from build123d import *
from OCP.BRepFilletAPI import BRepFilletAPI_MakeChamfer

# Parameters (mm, degrees)
CROQUIS2_W              = 16
CROQUIS2_H              = 23
SALIENTE_EXTRUIR1_DEPTH = 6
CORTAR_EXTRUIR1_DEPTH   = 3
CHAFL_N2_SIZE           = 3
CHAFL_N2_SIZE2          = 3.575260778
REDONDEO1_R             = 10
CHAFL_N1_SIZE           = 1
CROQUIS4_W              = 16
CROQUIS4_H              = 7
CORTAR_EXTRUIR2_DEPTH   = 1
SALIENTE_EXTRUIR2_DEPTH = 7
MATRIZL1_COUNT          = 8
MATRIZL1_PITCH          = 2


with BuildPart() as part:
    # Croquis2 → Saliente-Extruir1 (new body)
    with BuildSketch(Plane(origin=(0, 0, 0), x_dir=(-1, 0, 0), z_dir=(0, 0, -1))):
        with Locations((-8, 11.5)):
            Rectangle(CROQUIS2_W, CROQUIS2_H)
        with BuildLine():
            Line((-9.977670702, 6.125), (-9.977670702, 4.875))
            Line((-9.977670702, 4.875), (-9.124878317, 4.159422225))
            ThreePointArc((-9.124878317, 4.159422225), (-6.25, 5.5), (-9.124878317, 6.840577775))
            Line((-9.124878317, 6.840577775), (-9.977670702, 6.125))
        make_face(mode=Mode.SUBTRACT)
        with BuildLine():
            Line((-9.977670702, 18.125), (-9.977670702, 16.875))
            Line((-9.977670702, 16.875), (-9.124878317, 16.159422225))
            ThreePointArc((-9.124878317, 16.159422225), (-6.25, 17.5), (-9.124878317, 18.840577775))
            Line((-9.124878317, 18.840577775), (-9.977670702, 18.125))
        make_face(mode=Mode.SUBTRACT)
    extrude(amount=SALIENTE_EXTRUIR1_DEPTH)

    # Croquis3 → Cortar-Extruir1 (cut)
    with BuildSketch(Plane(origin=(-8, 0, 0), x_dir=(-1, 0, 0), z_dir=(0, 0, -1))):
        with BuildLine():
            Line((-19.864348845, 6.5), (-19.864348845, 4.5))
            Line((-19.864348845, 4.5), (-18.089059731, 3.01035556))
            ThreePointArc((-18.089059731, 3.01035556), (-12.75, 5.5), (-18.089059731, 7.98964444))
            Line((-18.089059731, 7.98964444), (-19.864348845, 6.5))
        make_face()
        with BuildLine():
            Line((-19.864348845, 18.5), (-18.089059731, 19.98964444))
            ThreePointArc((-18.089059731, 19.98964444), (-12.75, 17.5), (-18.089059731, 15.01035556))
            Line((-18.089059731, 15.01035556), (-19.864348845, 16.5))
            Line((-19.864348845, 16.5), (-19.864348845, 18.5))
        make_face()
    extrude(amount=CORTAR_EXTRUIR1_DEPTH, mode=Mode.SUBTRACT)

    # Chaflán2: one chamfer whose edges measure the first distance from different faces: ONE call of the kernel's chamfer builder (chamfer() names one face for all edges)
    chafl_n2_edges_1 = [part.edges().sort_by_distance(p)[0] for p in [
        (16, 23, -3),
        (16, 0, -3),
    ]]
    chafl_n2_side_1 = [part.faces().sort_by_distance(p)[0] for p in [
        (16, 11.5, -3),
    ]]
    chafl_n2_edges_2 = [part.edges().sort_by_distance(p)[0] for p in [
        (0, 23, -3),
        (0, 0, -3),
    ]]
    chafl_n2_side_2 = [part.faces().sort_by_distance(p)[0] for p in [
        (0, 11.5, -3),
    ]]
    chafl_n2 = BRepFilletAPI_MakeChamfer(part.part.solid().wrapped)
    for e in chafl_n2_edges_1:
        chafl_n2.Add(CHAFL_N2_SIZE, CHAFL_N2_SIZE2, e.wrapped, chafl_n2_side_1[0].wrapped)  # the first distance lies on this face
    for e in chafl_n2_edges_2:
        chafl_n2.Add(CHAFL_N2_SIZE, CHAFL_N2_SIZE2, e.wrapped, chafl_n2_side_2[0].wrapped)  # the first distance lies on this face
    add(Compound.cast(chafl_n2.Shape()), mode=Mode.REPLACE)

    # Redondeo1
    redondeo1_edges = [part.edges().sort_by_distance(p)[0] for p in [
        (3.575260778, 23, -3),
        (12.424739222, 23, -3),
        (3.575260778, 0, -3),
        (12.424739222, 0, -3),
    ]]
    fillet(redondeo1_edges, radius=REDONDEO1_R)

    # Chaflán1
    chafl_n1_edges = [part.edges().sort_by_distance(p)[0] for p in [
        (8, 0, 0),
        (8, 23, 0),
        (0.393543512, 20.330222216, 0),
        (15.606456488, 2.669777784, 0),
        (3.794761687, 22.396926208, 0),
        (12.205238313, 22.396926208, 0),
        (12.205238313, 0.603073792, 0),
        (3.794761687, 0.603073792, 0),
        (16, 11.5, 0),
        (0, 11.5, 0),
        (0.393543512, 2.669777784, 0),
        (15.606456488, 20.330222216, 0),
    ]]
    chamfer(chafl_n1_edges, length=CHAFL_N1_SIZE)

    # Croquis4 → Cortar-Extruir2 (cut)
    with BuildSketch(Plane(origin=(0, 0, -6), x_dir=(-1, 0, 0), z_dir=(0, 0, -1))):
        with Locations((-8, 11.5)):
            Rectangle(CROQUIS4_W, CROQUIS4_H)
    extrude(amount=-CORTAR_EXTRUIR2_DEPTH, mode=Mode.SUBTRACT)

    # Croquis5 → Saliente-Extruir2 (add)
    with BuildSketch(Plane(origin=(0, 8, 0), x_dir=(1, 0, 0), z_dir=(0, 1, 0))):
        Polygon((0, 5), (0.839099631, 6), (1.25, 6), (1.25, 5), align=None)
    saliente_extruir2 = extrude(amount=SALIENTE_EXTRUIR2_DEPTH)

    # MatrizL1: Saliente-Extruir2 ×8
    with Locations(*[(i * MATRIZL1_PITCH, 0, 0) for i in range(1, MATRIZL1_COUNT)]):
        add(saliente_extruir2)


solid = part.part
Input: part model. Units: mm. Frame: model coordinates. A direction names the side the tool comes from. Coordinates: 2 decimals unless noted, no trailing zeros. Loops run counter-clockwise (first coordinate to the right, second up) from the corner with the lowest first, then second, coordinate; pieces in that order, holes last. Notation, with made-up numbers: (62, 8) - (79, 8) arc R35 cw to (79, 41) - close; hole circle Ø10 at (64.5, 2.25). An arc over 180 degrees is marked (long way). Answer in a Markdown table with one row per item. Add a question column.
Item 1: Line query: line 1 along Y through (x, z) = (8, -4.2); line 2 along Y through (x, z) = (8, -1.75); line 3 along X through (y, z) = (5.5, -1.5). Output: solid intervals per line, ascending. Write a range as [from, to].
Item 2: Section query D-D on z = -5.5. State how many separate pieces and enclosed holes the cut face has, then the cut area to 3 significant figures.
Item 3: Access query for faces 5 (the flat face through (0, 11, -3)), 6 (the flat face through (13.9, 8, -5.6)), 7 (the cylindrical face through (4.75, 17.6, -1.48)). Directions: +Z, -Z, +X, -X, +Y, -Y. A direction counts if a zero-diameter tool reaches every point of the face in a straight line with its end or side. Return the directions, or none.
Item 4: Section query B-B on z = -2.25. Return the cut outline in (x, y), then the cut area to 3 significant figures.
Item 5: Contact query for flat-ended pins moving along their axis: P1, Ø1, axis at x = 12.5, z = -3, coming from the -Y side; P2, Ø2, axis at x = 12.5, z = -3.5, coming from the +Y side; P3, Ø0.6, axis at x = 15.5, z = -5.5, coming from the -Y side. Output: stop coordinate, or through.
Item 6: Section query C-C on z = -3.5. Return the cut outline in (x, y) (3 decimals).
Item 7: Section query A-A on y = 5.5. Return the cut outline in (x, z).
Item 8: Mould query, pull axis Y, two halves, no side actions, for faces 1 (the flat face through (0.2, 8, -5.7)), 2 (the flat face through (8.41, 11.45, -5.49)), 3 (the cylindrical face through (3.8, 22.4, -3.5)), 4 (the conical face through (4.045, 1.155, -0.396)). Classes: released by +Y, released by -Y, zero draft, split by the parting line, or undercut.
Recorded:
| question | item | result |
|---|---|---|
| 1 | line 1 | [0, 3.75], [7.25, 15.75], [19.25, 23] |
| 1 | line 2 | [0, 2.25], [8.75, 14.25], [20.75, 23] |
| 1 | line 3 | [0, 4.75], [11.86, 16] |
| 2 | separate pieces | 1 |
| 2 | enclosed holes | 9 |
| 2 | area | 255 mm^2 |
| 3 | face 5 | +Z, -Z, -X, +Y, -Y |
| 3 | face 6 | -Z |
| 3 | face 7 | +Z |
| 4 | outline | (0, 3) - (0.79, 2.34) arc R10 ccw to (7.21, 0) - (8.79, 0) arc R10 ccw to (15.21, 2.34) - (16, 3) - (16, 20) - (15.21, 20.66) arc R10 ccw to (8.79, 23) - (7.21, 23) arc R10 ccw to (0.79, 20.66) - (0, 20) - close; hole (10.09, 3.01) - (11.86, 4.5) - (11.86, 6.5) - (10.09, 7.99) arc R3.25 ccw (long way) to start; hole (10.09, 15.01) - (11.86, 16.5) - (11.86, 18.5) - (10.09, 19.99) arc R3.25 ccw (long way) to start |
| 4 | area | 270 mm^2 |
| 5 | P1 | y = 0.53 |
| 5 | P2 | y = 22.62 |
| 5 | P3 | y = 2.33 |
| 6 | outline | (0, 3) - (0.787, 2.34) arc R10 ccw to (7.215, 0) - (8.785, 0) arc R10 ccw to (15.213, 2.34) - (16, 3) - (16, 20) - (15.213, 20.66) arc R10 ccw to (8.785, 23) - (7.215, 23) arc R10 ccw to (0.787, 20.66) - (0, 20) - close; hole (9.125, 4.159) - (9.978, 4.875) - (9.978, 6.125) - (9.125, 6.841) arc R1.75 ccw (long way) to start; hole (9.125, 16.159) - (9.978, 16.875) - (9.978, 18.125) - (9.125, 18.841) arc R1.75 ccw (long way) to start |
| 7 | outline | (0, -6) - (6.25, -6) - (6.25, -3) - (4.75, -3) - (4.75, 0) - (1, 0) - (0, -1) - close; (9.98, -6) - (16, -6) - (16, -1) - (15, 0) - (11.86, 0) - (11.86, -3) - (9.98, -3) - close |
| 8 | face 1 | undercut |
| 8 | face 2 | undercut |
| 8 | face 3 | released by +Y |
| 8 | face 4 | released by -Y |
